Build history of the part. All positions in model axes, mm. Face numbers are marked on the shaded views. A direction names the side the tool comes from. Give positions to 0.01 mm unless a question says otherwise; leave off trailing zeros. Write each loop counter-clockwise with the first axis right and the second up, starting at its lowest first coordinate (ties: lowest second). Pieces come first, ordered by that corner, then holes.
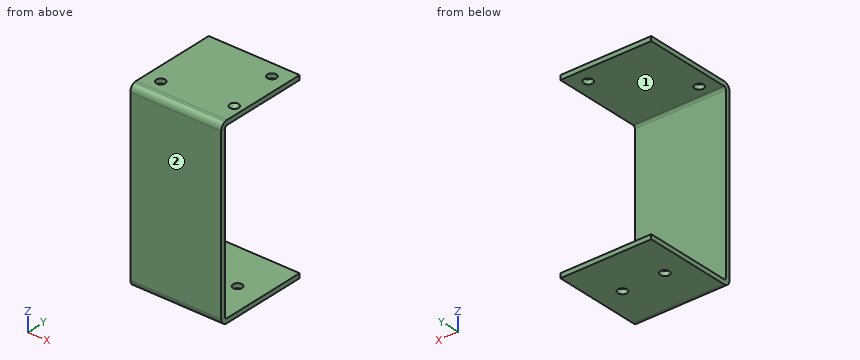
from build123d import *

# Parameters (mm, degrees)
SKETCH1_W                       = 30
SKETCH1_H                       = 118
SKETCH1_R                       = 1.5
BASE_FLANGE1_DEPTH              = 1.5
SKETCHED_BEND1_DEPTH            = 30
SKETCHED_BEND1_2_DEPTH          = 30
SKETCHED_START                  = -89.06902709
SKETCHED_BEND1_3_OUTLINE_R      = 1.5
SKETCHED_BEND1_3_DEPTH          = 1.5
SKETCHED_START_2                = -87.56902709
SKETCHED_BEND1_4_OUTLINE_R      = 1.5
SKETCHED_BEND1_4_DEPTH          = 59.56902709
F_3_0MM_PRESS_DOWEL_HOLE1_D     = 3
F_3_0MM_PRESS_DOWEL_HOLE1_DEPTH = 6
F_3_0MM_PRESS_DOWEL_HOLE1_TIP   = 0.901290929


with BuildPart() as part:
    # Base-Flange1: sheet metal written as solids
    # Sketch1 → Base-Flange1 (new body)
    with BuildSketch(Plane(origin=(0, 0, 0), x_dir=(1, 0, 0), z_dir=(0, 1, 0))):
        with Locations((15, 59)):
            Rectangle(SKETCH1_W, SKETCH1_H)
        with Locations(Location((8, 103, 0), (0, 0, 270))):
            Circle(SKETCH1_R, mode=Mode.SUBTRACT)
        with Locations(Location((22, 103, 0), (0, 0, 270))):
            Circle(SKETCH1_R, mode=Mode.SUBTRACT)
        with Locations(Location((25, 5, 0), (0, 0, 270))):
            Circle(SKETCH1_R, mode=Mode.SUBTRACT)
        with Locations(Location((5, 25, 0), (0, 0, 270))):
            Circle(SKETCH1_R, mode=Mode.SUBTRACT)
    extrude(amount=-BASE_FLANGE1_DEPTH)

    # Sketched Bend1: read off the stored shape, not the designer's step
    # Sketched Bend1 outline → Sketched Bend1 (cut)
    with BuildSketch(Plane.YZ):
        with BuildLine():
            ThreePointArc((0, -88.944250946), (-1.086838938, -88.127591172), (-1.5, -86.83242709))
            Line((-1.5, -86.83242709), (-1.5, -118))
            Line((-1.5, -118), (0, -118))
            Line((0, -118), (0, -88.944250946))
        make_face()
        with BuildLine():
            Line((-1.5, 0), (-1.5, -31.16757291))
            ThreePointArc((-1.5, -31.16757291), (-1.086838938, -29.872408828), (0, -29.055749054))
            Line((0, -29.055749054), (0, 0))
            Line((0, 0), (-1.5, 0))
        make_face()
    extrude(amount=SKETCHED_BEND1_DEPTH, mode=Mode.SUBTRACT)

    # Sketched Bend1 2 outline → Sketched Bend1 2 (add)
    with BuildSketch(Plane.YZ):
        with BuildLine():
            Line((0, -86.83242709), (0, -88.944250946))
            ThreePointArc((0, -88.944250946), (0.363053267, -89.037612433), (0.7366, -89.06902709))
            Line((0.7366, -89.06902709), (29.56902709, -89.06902709))
            Line((29.56902709, -89.06902709), (29.56902709, -87.56902709))
            Line((29.56902709, -87.56902709), (0.7366, -87.56902709))
            ThreePointArc((0.7366, -87.56902709), (0.215745145, -87.353281945), (0, -86.83242709))
        make_face()
        with BuildLine():
            ThreePointArc((0.7366, -28.93097291), (0.363053267, -28.962387567), (0, -29.055749054))
            Line((0, -29.055749054), (0, -31.16757291))
            ThreePointArc((0, -31.16757291), (0.215745145, -30.646718055), (0.7366, -30.43097291))
            Line((0.7366, -30.43097291), (29.56902709, -30.43097291))
            Line((29.56902709, -30.43097291), (29.56902709, -28.93097291))
            Line((29.56902709, -28.93097291), (0.7366, -28.93097291))
        make_face()
    extrude(amount=SKETCHED_BEND1_2_DEPTH)

    # Sketched Bend1 3 outline → Sketched Bend1 3 (cut)
    with BuildSketch(Plane.XY.offset(SKETCHED_START)):
        with Locations((8, 14.56902709)):
            Circle(SKETCHED_BEND1_3_OUTLINE_R)
        with Locations((22, 14.56902709)):
            Circle(SKETCHED_BEND1_3_OUTLINE_R)
    extrude(amount=SKETCHED_BEND1_3_DEPTH, mode=Mode.SUBTRACT)

    # Sketched Bend1 4 outline → Sketched Bend1 4 (cut)
    with BuildSketch(Plane.XY.offset(SKETCHED_START_2)):
        with Locations((5, 4.56902709)):
            Circle(SKETCHED_BEND1_4_OUTLINE_R)
        with Locations((25, 24.56902709)):
            Circle(SKETCHED_BEND1_4_OUTLINE_R)
    extrude(amount=SKETCHED_BEND1_4_DEPTH, mode=Mode.SUBTRACT)

    # Ø3.0mm Press Dowel Hole1
    with Locations(Plane(origin=(257.525513363, 325.031359221, -22.93097291), x_dir=(-1, 0, 0), z_dir=(0, 0, 1))):
        with Locations((220.525513363, 156.531359221), (102.525513363, 181.531359221), (102.525513363, 271.531359221), (89.19270005, 226.531359221), (210.525513363, 317.793651488), (230.525513363, 317.793651488), (252.525513363, 320.462332131), (232.525513363, 300.462332131), (252.525513363, 132.600386311), (232.525513363, 152.600386311), (111.286271896, 136.531359221), (91.286271896, 136.531359221), (41.525513363, 196.432813402), (13.525513363, 196.432813402), (41.525513363, 138.767959221), (13.525513363, 138.767959221), (41.525513363, 256.62990504), (13.525513363, 256.62990504), (41.525513363, 314.294759221), (13.525513363, 314.294759221)):
            Hole(F_3_0MM_PRESS_DOWEL_HOLE1_D / 2, depth=F_3_0MM_PRESS_DOWEL_HOLE1_DEPTH)
            with Locations((0, 0, -(F_3_0MM_PRESS_DOWEL_HOLE1_DEPTH + F_3_0MM_PRESS_DOWEL_HOLE1_TIP / 2))):  # 118° drill point
                Cone(0, F_3_0MM_PRESS_DOWEL_HOLE1_D / 2, F_3_0MM_PRESS_DOWEL_HOLE1_TIP, mode=Mode.SUBTRACT)


solid = part.part
1. Drill centre lines: line 1 along Z through (x, y) = (1.75, 4); line 2 along Y through (x, z) = (2.5, -48); line 3 along Y through (x, z) = (5, -30.1). Where is each one in solid material? Low to high.
2. Saw through at D-D on z = -40.5. Give the cut face in (x, y).
3. Saw through at A-A on x = 8. Give the cut face in (y, z), plus the area to 4 significant figures.
4. 3-axis set-ups, long thin cutter, end or side, ignore diameter. For the marked faces 1 and 2: which of +Z, -Z, +X, -X, +Y, -Y reach the whole face in a straight line?
5. Saw through at B-B on y = 20. Give the cut face in (x, z).
6. Drop flat-ended pins along their axis: pin 1 (3 mm diameter, centred on x = 21.5, z = -51, fed in from +Y); pin 2 (2.5 mm diameter, centred on x = 22, y = 14.57, fed in from -Z). Give the stop position or say it passes through.
7. Saw through at C-C on x = 18.5. Give the cut face in (y, z), plus the area to 3 significant figures.
Outcome:
1. line 1: z = -89.07 to -87.57, -30.43 to -28.93
1. line 2: y = -1.5 to 0
1. line 3: y = -1.23 to 3.07, 6.07 to 29.57
2. outline: (0, -1.5) - (30, -1.5) - (30, 0) - (0, 0) - close
3. outline: (-1.5, -86.83) arc R2.24 ccw to (0.74, -89.07) - (13.07, -89.07) - (13.07, -87.57) - (0.74, -87.57) arc R0.74 cw to (0, -86.83) - (0, -31.17) arc R0.74 cw to (0.74, -30.43) - (29.57, -30.43) - (29.57, -28.93) - (0.74, -28.93) arc R2.24 ccw to (-1.5, -31.17) - close; (16.07, -89.07) - (29.57, -89.07) - (29.57, -87.57) - (16.07, -87.57) - close
3. area: 172.5 mm2
4. face 1: +X, -X, +Y
4. face 2: +Z, -Z, +X, -X, -Y
5. outline: (0, -89.07) - (30, -89.07) - (30, -87.57) - (0, -87.57) - close; (0, -30.43) - (30, -30.43) - (30, -28.93) - (0, -28.93) - close
6. pin 1: stops at y = 0
6. pin 2: stops at z = -30.43
7. outline: (-1.5, -86.83) arc R2.24 ccw to (0.74, -89.07) - (29.57, -89.07) - (29.57, -87.57) - (0.74, -87.57) arc R0.74 cw to (0, -86.83) - (0, -31.17) arc R0.74 cw to (0.74, -30.43) - (29.57, -30.43) - (29.57, -28.93) - (0.74, -28.93) arc R2.24 ccw to (-1.5, -31.17) - close
7. area: 177 mm2
